Verification items for the finished model (mm, model axes). A direction names the side the tool comes from. Coordinates: 2 decimals unless noted, no trailing zeros. Order: outer loops, then holes, each group sorted by start corner. A loop starts at its lowest first (then second) coordinate and runs counter-clockwise, first axis right, second up. Notation, with made-up numbers: M -14.5,13 L -9.5,13 A28 cw -9.5,40 Z; hole C 55.25,-32.5 d8. An arc over 180 degrees is marked long. Return JSON: item names as keys, results as strings. Group by question number.
1. Section check D-D, the plane y = 5. Record the cut outline in (x, z) (3 decimals), plus the area to 3 significant figures.
2. Mould release check, pull along X, two halves, no side actions. Record for faces 5 (the cylindrical face through (3, 1, 0)), 6 (the flat face through (0, 7, 3.75)), 7 (the cylindrical face through (4.126, 6.76, -2.394)), 8 (the cylindrical face through (2.394, 6.76, 4.126)): +X half, -X half, draft (parallel to the pull), parting line (faces both ways), or undercut.
3. Section check C-C, the plane y = 6.75. Give the number of separate pieces and of enclosed holes in the cut face, plus the area to 3 significant figures.
4. Gauge pin test, flat ends, axial feed: pin 1 (5 mm diameter, centred on x = -7, z = 6.5, fed in from +Y); pin 2 (1.6 mm diameter, centred on y = 7, z = 0.5, fed in from +X); pin 3 (3 mm diameter, centred on x = 4.5, y = 5.5, fed in from -Z). Record the tip position at first contact, or that the pin passes through.
5. Set-up check for faces 1 (the cylindrical face through (4.106, 6.76, 2.374)), 2 (the cylindrical face through (2.374, 6.76, -4.106)), 3 (the cylindrical face through (2.374, 6.76, 5.894)), 4 (the cylindrical face through (-2.394, 6.76, 5.874)): record each of +Z, -Z, +X, -X, +Y, -Y from which the full face is reachable in a straight line by a thin tool's end or side.
6. Material ranges on line 1 along Z through (x, y) = (0, 0.15) (3 decimals); line 2 along Z through (x, y) = (0, 4.55) (3 decimals); line 3 along Y through (x, z) = (2.5, 7.75), recorded low to high.
Autodesk Inventor part; units mm, degrees
ref_plane "YZ Plane" through (0, 0, 0) normal (1, 0, 0) x (0, 1, 0)
ref_plane "XZ Plane" through (0, 0, 0) normal (0, 1, 0) x (-1, 0, 0)
ref_plane "XY Plane" through (0, 0, 0) normal (0, 0, 1) x (1, 0, 0)
sketch "Sketch1" plane through (0, 0, 0) normal (0, 1, 0) x (-1, 0, 0)
  circle A0 centre (0, 0) radius 7.375
  circle A1 centre (0, 0) radius 1.75
  circle A2 centre (0, 0) radius 10
  circle A3 centre (0, 0) radius 3
  dimension "d0" = 14.75
  dimension "d1" = 3.5
  dimension "d2" = 20
  dimension "d7" = 6
extrude "Extrusion1" add sketch "Sketch1" along normal blind 6 contours A0 | A3
extrude "Extrusion2" add sketch "Sketch1" against normal blind 2 contours A0 | A2
sketch "Sketch2" plane through (0, 6, 0) normal (0, 1, 0) x (1, 0, 0)
  line L0 (3.75, -2.75) -> (6.25, -2.75)
  line L1 (6.25, -2.75) -> (6.25, 2.75)
  line L2 (6.25, 2.75) -> (3.75, 2.75)
  line L3 (3.75, 2.75) -> (3.75, -2.75)
  line L4 (3.75, -2.75) -> (6.25, 2.75) construction
  line L5 (6.25, -2.75) -> (3.75, 2.75) construction
  line L6 (-2.75, 3.75) -> (2.75, 3.75)
  line L7 (2.75, 3.75) -> (2.75, 6.25)
  line L8 (2.75, 6.25) -> (-2.75, 6.25)
  line L9 (-2.75, 6.25) -> (-2.75, 3.75)
  line L10 (-3.75, -2.75) -> (-3.75, 2.75)
  line L11 (-3.75, 2.75) -> (-6.25, 2.75)
  line L12 (-6.25, 2.75) -> (-6.25, -2.75)
  line L13 (-6.25, -2.75) -> (-3.75, -2.75)
  line L14 (2.75, -3.75) -> (-2.75, -3.75)
  line L15 (-2.75, -3.75) -> (-2.75, -6.25)
  line L16 (-2.75, -6.25) -> (2.75, -6.25)
  line L17 (2.75, -6.25) -> (2.75, -3.75)
  point P0 (0, 0)
  point P1 (5, 0)
  dimension "d10" = 5.5
  dimension "d11" = 2.5
  dimension "d12" = 5
  dimension "d13" = 0
  dimension "d16" = 360
extrude "Extrusion4" add sketch "Sketch2" along normal blind 1.5
fillet "Fillet1" radius 1.25 16 edges at (6.25, 6.75, -2.75) (3.75, 6.75, -2.75) (6.25, 6.75, 2.75) (3.75, 6.75, 2.75) (2.75, 6.75, 3.75) (2.75, 6.75, 6.25) (-2.75, 6.75, 6.25) (-2.75, 6.75, 3.75) (-3.75, 6.75, 2.75) (-6.25, 6.75, 2.75) (-6.25, 6.75, -2.75) (-3.75, 6.75, -2.75) (-2.75, 6.75, -6.25) (-2.75, 6.75, -3.75) (2.75, 6.75, -6.25) (2.75, 6.75, -3.75)
fillet "Fillet2" radius 0.5 3 edges at (10, -2, 0) (10, 0, 0) (3, -2, 0)
extrude "Extrusion5" cut sketch "Sketch1" along normal blind 3 contours A3
equation "\"d0\" = ShaftDiameter"
equation "\"d1\" = HoleDiameter"
equation "\"d2\" = CapDiameter"
equation "\"d3\" = ShaftLength"
equation "\"d5\" = CapLength"
equation "\"d18\" = TabLength"
equation "\"CapDiameter\" = 20"
equation "\"HoleDiameter\" = 3.5"
equation "\"ShaftLength\" = FEMUR_HEIGHT"
equation "\"CapLength\" = 2"
equation "\"HoleLength\" = 5"
equation "\"TabLength\" = 1.5"
properties part number "AxleCap"
Answers follow:
{
 "1": {"outline": "C 0,0 d14.75; hole C 0,0 d3.5", "area": "161 mm^2"},
 "2": {"face 5": "undercut", "face 6": "draft", "face 7": "undercut", "face 8": "+X half"},
 "3": {"separate pieces": "4", "enclosed holes": "0", "area": "49.6 mm^2"},
 "4": {"pin 1": "y = 6", "pin 2": "x = 6.25", "pin 3": "z = -6.74"},
 "5": {"face 1": "+Z, +Y", "face 2": "+X, +Y", "face 3": "+Z, +X, +Y", "face 4": "+Z, -X, +Y"},
 "6": {"line 1": "-7.375 to -3, 3 to 7.375", "line 2": "-7.375 to -1.75, 1.75 to 7.375", "line 3": "-2 to 0"}
}
